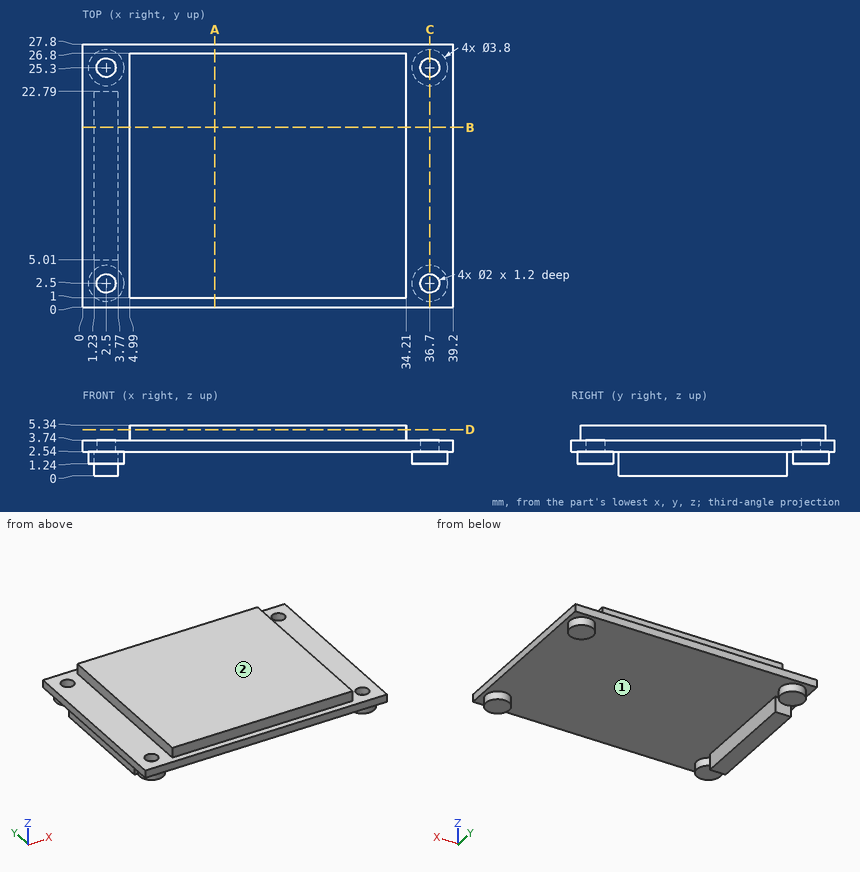
Input: dimensioned drawing with shaded views. Units: mm. Origin: part minimum x, y, z. Coordinates: 2 decimals unless noted, no trailing zeros. Order: outer loops, then holes, each group sorted by start corner. A loop starts at its lowest first (then second) coordinate and runs counter-clockwise, first axis right, second up. Notation, with made-up numbers: (-22, -21.75) - (12, -21.75) arc R13 ccw to (12, -16.75) - close; hole circle Ø1 at (-21, 84.25). An arc over 180 degrees is marked (long way). Put each result on its own line as item: value.
1. Cut plane C-C on x = 36.7. Return the cut outline in (y, z).
Report:
outline: (0, 2.54) - (0.6, 2.54) - (0.6, 1.24) - (4.4, 1.24) - (4.4, 2.54) - (23.4, 2.54) - (23.4, 1.24) - (27.2, 1.24) - (27.2, 2.54) - (27.8, 2.54) - (27.8, 3.74) - (26.3, 3.74) - (26.3, 2.54) - (24.3, 2.54) - (24.3, 3.74) - (3.5, 3.74) - (3.5, 2.54) - (1.5, 2.54) - (1.5, 3.74) - (0, 3.74) - close
2. Cut plane D-D on z = 4.85. Return the cut outline in (x, y), then the cut area to 3 significant figures.
Report:
outline: (4.99, 1) - (34.21, 1) - (34.21, 26.8) - (4.99, 26.8) - close
area: 754 mm2
3. Cut plane B-B on y = 19. Return the cut outline in (x, z), then the cut area to 3 significant figures.
Report:
outline: (0, 2.54) - (1.23, 2.54) - (1.23, 0) - (3.77, 0) - (3.77, 2.54) - (39.2, 2.54) - (39.2, 3.74) - (34.21, 3.74) - (34.21, 5.34) - (4.99, 5.34) - (4.99, 3.74) - (0, 3.74) - close
area: 100 mm2
4. Cut plane A-A on x = 14. Return the cut outline in (y, z).
Report:
outline: (0, 2.54) - (27.8, 2.54) - (27.8, 3.74) - (26.8, 3.74) - (26.8, 5.34) - (1, 5.34) - (1, 3.74) - (0, 3.74) - close
5. Draft query along X for the marked faces 1 and 2. Return one class per face: pulls with the +X half, pulls with the -X half, needs draft (parallel to the pull), parting line crosses it, or undercut.
Report:
face 1: undercut
face 2: needs draft
6. Contact query for flat-ended pins moving along their axis: pin 1 Ø1.9 at (x, y) = (3.5, 26) entering from -Z; pin 2 Ø0.6 at (x, y) = (36.5, 25.5) entering from +Z; pin 3 Ø0.8 at (x, z) = (2, 1) entering from +Y. Output: stop coordinate, or through.
Report:
pin 1: stops at z = 1.24
pin 2: stops at z = 2.54
pin 3: stops at y = 27.19
7. Line query: line 1 along X through (y, z) = (25.3, 3.15); line 2 along Y through (x, z) = (2.5, 3.3); line 3 along X through (y, z) = (24.75, 3.4). Output: solid intervals per line, ascending.
Report:
line 1: x = 0 to 1.5, 3.5 to 35.7, 37.7 to 39.2
line 2: y = 0 to 1.5, 3.5 to 24.3, 26.3 to 27.8
line 3: x = 0 to 1.66, 3.34 to 35.86, 37.54 to 39.2
